The figure shows three views and two pictorial views of one solid part (mm, origin at its lowest corner). Answer the questions. A direction names the side the tool comes from. Coordinates: 2 decimals unless noted, no trailing zeros. Loops run counter-clockwise (first coordinate to the right, second up) from the corner with the lowest first, then second, coordinate; pieces in that order, holes last. Notation, with made-up numbers: (46.25, -24) -> (94.25, -24) arc R17 cw to (94.25, -9) -> close; hole circle Ø10 at (72, 21.25). An arc over 180 degrees is marked (long way). Answer in a Markdown table with one row per item.
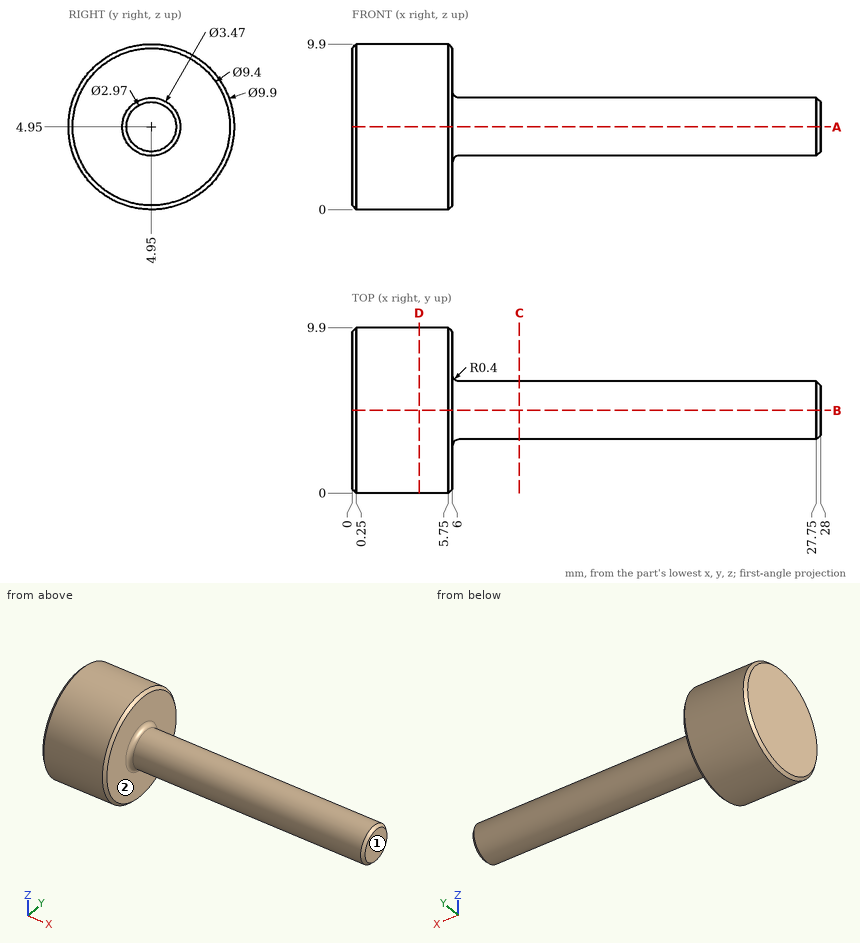
Item 1: Flat-ended cylindrical pins translate along their axes: pin 1 Ø3 at (x, y) = (14.5, 9) entering from +Z; pin 2 Ø4 at (x, z) = (22, 3) entering from +Y (3 decimals). Find the tip coordinate at first contact, or state that the pin passes through.
Findings below:
| item | result |
|---|---|
| pin 1 | passes through |
| pin 2 | stops at y = 6.685 |
Item 2: Find the intervals of material crossed by probe 1 along Y at (x, z) = (25.5, 5); probe 2 along X at (y, z) = (0.5, 4.5); probe 3 along X at (y, z) = (4.75, 6.75), in increasing order.
Findings below:
| item | result |
|---|---|
| probe 1 | y = 3.22 to 6.68 |
| probe 2 | x = 0 to 6 |
| probe 3 | x = 0 to 6.17 |
Item 3: A tool of negligible diameter and unlimited length cuts with its end or side. For the marked faces 1 and 2, from which of +Z, -Z, +X, -X, +Y, -Y can it reach the whole face along a straight path? Write none if from no direction.
Findings below:
| item | result |
|---|---|
| face 1 | +Z, -Z, +X, +Y, -Y |
| face 2 | +X |
Item 4: A cutting plane is placed at C-C, the plane x = 10. Determine the outline of the cut face in (y, z) (3 decimals), plus the area to 3 significant figures.
Findings below:
| item | result |
|---|---|
| outline | circle Ø3.47 at (4.95, 4.95) |
| area | 9.46 mm2 |
Item 5: A cutting plane is placed at D-D, the plane x = 4. Determine the outline of the cut face in (y, z).
Findings below:
| item | result |
|---|---|
| outline | circle Ø9.9 at (4.95, 4.95) |
Item 6: A cutting plane is placed at A-A, the plane z = 4.95. Determine the outline of the cut face in (x, y) (3 decimals), plus the area to 3 significant figures.
Findings below:
| item | result |
|---|---|
| outline | (0, 0.25) -> (0.25, 0) -> (5.75, 0) -> (6, 0.25) -> (6, 2.815) arc R0.4 cw to (6.4, 3.215) -> (27.75, 3.215) -> (28, 3.465) -> (28, 6.435) -> (27.75, 6.685) -> (6.4, 6.685) arc R0.4 cw to (6, 7.085) -> (6, 9.65) -> (5.75, 9.9) -> (0.25, 9.9) -> (0, 9.65) -> close |
| area | 136 mm2 |
